from build123d import *

# Parameters (mm, degrees)
SKETCH1_W           = 200
SKETCH1_H           = 190
BOSS_EXTRUDE1_DEPTH = 10
SKETCH2_W           = 20
SKETCH2_H           = 7
SKETCH2_W_2         = 16
SKETCH2_H_2         = 6
CUT_EXTRUDE1_DEPTH  = 10
SKETCH4_R           = 3
CUT_EXTRUDE2_DEPTH  = 10
SKETCH5_R           = 3
CUT_EXTRUDE3_DEPTH  = 10


with BuildPart() as part:
    # Sketch1 → Boss-Extrude1 (new body)
    with BuildSketch(Plane(origin=(0, 0, 0), x_dir=(1, 0, 0), z_dir=(0, 1, 0))):
        with Locations((100, 95)):
            Rectangle(SKETCH1_W, SKETCH1_H)
    extrude(amount=BOSS_EXTRUDE1_DEPTH)

    # Sketch2 → Cut-Extrude1 (cut)
    with BuildSketch(Plane(origin=(0, 0, -190), x_dir=(-1, 0, 0), z_dir=(0, 0, -1))):
        with Locations((-128, 5.5)):
            Rectangle(SKETCH2_W, SKETCH2_H)
        with Locations((-72, 5.5)):
            Rectangle(SKETCH2_W, SKETCH2_H)
        with Locations((-30, 5)):
            Rectangle(SKETCH2_W_2, SKETCH2_H_2)
        with Locations((-170, 5)):
            Rectangle(SKETCH2_W_2, SKETCH2_H_2)
    extrude(amount=-CUT_EXTRUDE1_DEPTH, mode=Mode.SUBTRACT)

    # Sketch4 → Cut-Extrude2 (cut)
    with BuildSketch(Plane(origin=(0, 0, 0), x_dir=(-1, 0, 0), z_dir=(0, -1, 0))):
        with Locations(Location((-10, 142.5, 0), (0, 0, 90))):
            Circle(SKETCH4_R)
        with Locations(Location((-10, 95, 0), (0, 0, 90))):
            Circle(SKETCH4_R)
        with Locations(Location((-190, 95, 0), (0, 0, 270))):
            Circle(SKETCH4_R)
        with Locations(Location((-190, 142.5, 0), (0, 0, 270))):
            Circle(SKETCH4_R)
    extrude(amount=-CUT_EXTRUDE2_DEPTH, mode=Mode.SUBTRACT)

    # Sketch5 → Cut-Extrude3 (cut)
    with BuildSketch(Plane(origin=(0, 10, 0), x_dir=(1, 0, 0), z_dir=(0, 1, 0))):
        with Locations(Location((100, 20, 0), (0, 0, 270))):
            Circle(SKETCH5_R)
    extrude(amount=-CUT_EXTRUDE3_DEPTH, mode=Mode.SUBTRACT)


solid = part.part
Design review of the part built by this model. Coordinates are the model's own, in mm. A direction names the side the tool comes from. Round coordinates to 2 decimals unless told otherwise and drop trailing zeros. Write each loop counter-clockwise with the first axis right and the second up, starting at its lowest first coordinate (ties: lowest second). Pieces come first, ordered by that corner, then holes. Notation, with made-up numbers: (35.5, 37) -> (44.5, 37) arc R17 cw to (44.5, 46) -> close; hole circle Ø1 at (-27, 19). An arc over 180 degrees is marked (long way). One line per question, with ' | ' between items.
(1) Draft analysis for pull direction Z (two halves, no side actions). For faces 1 (the cylindrical face through (187.47, 4.93, -140.89)), 2 (the flat face through (30, 5, -180)), 3 (the flat face through (200, 5, -94)), state which applies: released by +Z, released by -Z, zero draft, split by the parting line, or undercut.
Result sheet:
face 1: undercut | face 2: released by -Z | face 3: zero draft
(2) Machinability: for faces 4 (the flat face through (178, 5, -185)), 5 (the cylindrical face through (10.9, 4.93, -145.36)), which of the approach directions +Z, -Z, +X, -X, +Y, -Y give a long, thin tool a straight path to every point of the face, cutting with its end or side? Answer none if there is none.
Result sheet:
face 4: -Z | face 5: +Y, -Y
(3) Take a section at C-C, the plane x = 10. State the section outline as (y, z) points, and give its area (3 significant figures).
Result sheet:
outline: (0, -190) -> (10, -190) -> (10, -145.5) -> (0, -145.5) -> close; (0, -139.5) -> (10, -139.5) -> (10, -98) -> (0, -98) -> close; (0, -92) -> (10, -92) -> (10, 0) -> (0, 0) -> close | area: 1,780 mm2
(4) Take a section at B-B, the plane z = -20. State the section outline as (x, y) points, and give its area (3 significant figures).
Result sheet:
outline: (0, 0) -> (97, 0) -> (97, 10) -> (0, 10) -> close; (103, 0) -> (200, 0) -> (200, 10) -> (103, 10) -> close | area: 1,940 mm2
(5) Insertion check: P1, Ø3.5, axis at x = 131, y = 5.5, coming from the -Z side. The pin has a flat end and moves straight along its axis. Give the tip position at first contact, or say it passes through.
Result sheet:
P1: z = -180
(6) Take a section at A-A, the plane x = 100. State the section outline as (y, z) points, and give its area (3 significant figures).
Result sheet:
outline: (0, -190) -> (10, -190) -> (10, -23) -> (0, -23) -> close; (0, -17) -> (10, -17) -> (10, 0) -> (0, 0) -> close | area: 1,840 mm2
(7) Take a section at D-D, the plane z = -142.5. State the section outline as (x, y) points, and give its area (3 significant figures).
Result sheet:
outline: (0, 0) -> (7, 0) -> (7, 10) -> (0, 10) -> close; (13, 0) -> (187, 0) -> (187, 10) -> (13, 10) -> close; (193, 0) -> (200, 0) -> (200, 10) -> (193, 10) -> close | area: 1,880 mm2
(8) Wall thickness on line 1 (X direction, y = 3.75, z = -142.5); line 2 (Z direction, x = 190, y = 3); line 3 (X direction, y = 3, z = -20): over which ranges is each line inside the solid? List them lowest first. Write a range as [from, to].
Result sheet:
line 1: [0, 7], [13, 187], [193, 200] | line 2: [-190, -145.5], [-139.5, -98], [-92, 0] | line 3: [0, 97], [103, 200]
